Verification items for the finished model (mm, model axes). A direction names the side the tool comes from. Give positions to 0.01 mm unless a question says otherwise; leave off trailing zeros.
(1) Access from +Z, -Z, +X, -X, +Y, -Y to the whole of each face (thin tool, end or side, straight path). Record for faces 4 (the face through (-1, 0, -1)), 5 (the face through (-28, 19.225, -61)), 6 (the face through (-2, 3.175, 8)).
(2) Sectioned sample at A-A on z = 19.05. Count the separate pieces of the cut face and the enclosed holes in it, plus the area to 3 significant figures.
(3) Mould release check, pull along Z, two halves, no side actions. Record for faces 1 (the face through (-28, 22.225, 55)), 2 (the face through (-13.77, 8, 61.99)), 3 (the face through (-18.136, 1.61, 17.617)): pulls with the +Z half, pulls with the -Z half, needs draft (parallel to the pull), parting line crosses it, or undercut.
(4) Scan lines: L1, parallel to X at y = 4, z = 9.5; L2, parallel to Z at x = -7, y = 20.25; L3, parallel to Y at x = -34, z = 21.5 (3 decimals). Record each from-to range of solid material in increasing order.
(5) Gauge pin test, flat ends, axial feed: pin 1 (1.5 mm diameter, centred on y = 13.5, z = -17.5, fed in from -X); pin 2 (6.5 mm diameter, centred on x = -3, z = -2.5, fed in from +Y) (3 decimals); pin 3 (3 mm diameter, centred on y = 14.5, z = -4, fed in from -X); pin 4 (3 mm diameter, centred on x = 0, z = 70.1, fed in from +Y) (3 decimals). Record the tip position at first contact, or that the pin passes through.
```python
from build123d import *

# Parameters (mm, degrees)
SKETCH1_R             = 63.5
SKETCH1_R_2           = 60.690000065
BOSS_EXTRUDE1_DEPTH   = 22.225
SKETCH3_R             = 63.5
BOSS_EXTRUDE2_DEPTH   = 3.175
SKETCH8_R             = 13
SKETCH8_R_2           = 11
BOSS_EXTRUDE4_DEPTH   = 7
SKETCH10_R            = 74.095000033
SKETCH10_R_2          = 63.5
BOSS_EXTRUDE5_DEPTH   = 3
M3X0_5_TAPPED_HOLE1_D = 2.5
CIRPATTERN2_COUNT     = 8
SKETCH16_R            = 8
CUT_EXTRUDE1_DEPTH    = 1.5
FILLET1_R             = 2
FILLET2_R             = 3
SKETCH19_R            = 1.7
CUT_EXTRUDE2_DEPTH    = 4.175


with BuildPart() as part:
    # Sketch1 → Boss-Extrude1 (new body)
    with BuildSketch(Plane(origin=(0, 0, 0), x_dir=(1, 0, 0), z_dir=(0, 1, 0))):
        Circle(SKETCH1_R)
        Circle(SKETCH1_R_2, mode=Mode.SUBTRACT)
    extrude(amount=BOSS_EXTRUDE1_DEPTH)

    # Sketch3 → Boss-Extrude2 (add)
    with BuildSketch(Plane(origin=(0, 0, 0), x_dir=(1, 0, 0), z_dir=(0, 1, 0))):
        Circle(SKETCH3_R)
    extrude(amount=BOSS_EXTRUDE2_DEPTH)

    # Sketch8 → Boss-Extrude4 (add)
    with BuildSketch(Plane(origin=(0, 3.175, 0), x_dir=(1, 0, 0), z_dir=(0, 1, 0))):
        Circle(SKETCH8_R)
        Circle(SKETCH8_R_2, mode=Mode.SUBTRACT)
    extrude(amount=BOSS_EXTRUDE4_DEPTH)

    # Sketch10 → Boss-Extrude5 (add)
    with BuildSketch(Plane(origin=(0, 22.225, 0), x_dir=(1, 0, 0), z_dir=(0, 1, 0))):
        Circle(SKETCH10_R)
        Circle(SKETCH10_R_2, mode=Mode.SUBTRACT)
    extrude(amount=-BOSS_EXTRUDE5_DEPTH)

    # M3x0.5 Tapped Hole1 (through all)
    with Locations(Plane(origin=(0, 22.225, 0), x_dir=(1, 0, 0), z_dir=(0, 1, 0))):
        with Locations((-70.1, 0)):
            m3x0_5_tapped_hole1 = Hole(M3X0_5_TAPPED_HOLE1_D / 2)

    # CirPattern2: M3x0.5 Tapped Hole1 ×8 about axis
    cirpattern2_axis = Axis((0, 0, 0), (0, 1, 0))
    for i in range(1, CIRPATTERN2_COUNT):
        add(m3x0_5_tapped_hole1.rotate(cirpattern2_axis, i * 360 / CIRPATTERN2_COUNT), mode=Mode.SUBTRACT)

    # Sketch16 → Cut-Extrude1 (cut)
    with BuildSketch(Plane(origin=(0, 3.175, 0), x_dir=(1, 0, 0), z_dir=(0, 1, 0))):
        Circle(SKETCH16_R)
    extrude(amount=-CUT_EXTRUDE1_DEPTH, mode=Mode.SUBTRACT)

    # Fillet1
    fillet1_edges = [part.edges().sort_by_distance(p)[0] for p in [
        (-13, 3.175, 0),
    ]]
    fillet(fillet1_edges, radius=FILLET1_R)

    # Fillet2
    fillet2_edges = [part.edges().sort_by_distance(p)[0] for p in [
        (-63.5, 19.225, 0),
    ]]
    fillet(fillet2_edges, radius=FILLET2_R)

    # Sketch19 → Cut-Extrude2 (cut, through all)
    with BuildSketch(Plane(origin=(0, 3.175, 0), x_dir=(1, 0, 0), z_dir=(0, 1, 0))):
        with Locations((19.05, -19.05)):
            Circle(SKETCH19_R)
        with Locations((19.05, 19.05)):
            Circle(SKETCH19_R)
        with Locations((-19.05, -19.05)):
            Circle(SKETCH19_R)
        with Locations((-19.05, 19.05)):
            Circle(SKETCH19_R)
    extrude(amount=-CUT_EXTRUDE2_DEPTH, mode=Mode.SUBTRACT)


solid = part.part
```
Ans:
1. face 4: +Z, -Z, +X, -X, -Y
1. face 5: -Y
1. face 6: +Y
2. separate pieces: 3
2. enclosed holes: 0
2. area: 546 mm2
3. face 1: needs draft
3. face 2: parting line crosses it
3. face 3: undercut
4. L1: x = -62.79 to -59.94, -9.42 to -5.55, 5.55 to 9.42, 59.94 to 62.79
4. L2: z = -73.76 to -60.28, 60.28 to 73.76
4. L3: y = 0 to 3.175
5. pin 1: stops at x = -61.25
5. pin 2: stops at y = 1.675
5. pin 3: stops at x = -63.45
5. pin 4: stops at y = 22.225
